Autodesk Inventor part; units mm, degrees
ref_plane "YZ Plane" through (0, 0, 0) normal (1, 0, 0) x (0, 1, 0)
ref_plane "XZ Plane" through (0, 0, 0) normal (0, 1, 0) x (-1, 0, 0)
ref_plane "XY Plane" through (0, 0, 0) normal (0, 0, 1) x (1, 0, 0)
sketch "Sketch1" plane through (0, 0, 0) normal (1, 0, 0) x (0, 1, 0)
  line L0 (0, 0) -> (11.43, 0)
  line L1 (11.43, 0) -> (11.43, -28.575)
  line L2 (11.43, -28.575) -> (0, -28.575)
  line L3 (0, -28.575) -> (0, 0)
  line L4 (0, 0) -> (8.255, 0)
  line L5 (8.255, 0) -> (8.255, -25.4)
  line L6 (8.255, -25.4) -> (0, -25.4)
  line L7 (0, -25.4) -> (0, 0)
  dimension "d0" = 11.43
  dimension "d1" = 28.575
  dimension "d2" = 8.255
  dimension "d3" = 25.4
extrude "Extrusion1" add sketch "Sketch1" along normal blind 19.05 contours L0 L1 L2 L3 L6 L5
sketch "Sketch2" plane through (0, 11.43, 0) normal (0, 1, 0) x (1, 0, 0)
  line L0 (0, 28.575) -> (0, 0)
  line L1 (0, 0) -> (19.05, 0)
  line L2 (19.05, 28.575) -> (19.05, 0)
  line L3 (0, 28.575) -> (19.05, 28.575)
  point P0 (0, 0)
  point P1 (4.7625, 6.35)
  point P2 (14.2875, 6.35)
  dimension "d6" = 9.525
  dimension "d7" = 4.7625
  dimension "d8" = 28.575
  dimension "d31" = 19.05
  dimension "d33" = 6.35
  dimension "d34" = 6.35
hole "Hole1" at (4.7625, 11.43, -6.35) at (14.2875, 11.43, -6.35) direction (0, -1, 0) diameter 3.429 end through all
sketch "Sketch3" plane through (0, 0, -25.4) normal (0, 0, 1) x (1, 0, 0)
  line L0 (0, 0) -> (0, 8.255)
  line L1 (19.05, 0) -> (0, 0)
  line L2 (19.05, 8.255) -> (19.05, 0)
  line L3 (0, 8.255) -> (19.05, 8.255)
  point P0 (0, 0)
  point P1 (4.7625, 4.1275)
  point P2 (14.2875, 4.1275)
  dimension "d20" = 9.525
  dimension "d21" = 4.7625
  dimension "d22" = 4.1275
  dimension "d23" = 4.1275
  dimension "d32" = 19.05
  dimension "d35" = 8.255
hole "Hole2" at (4.7625, 4.1275, -25.4) at (14.2875, 4.1275, -25.4) direction (0, 0, -1) diameter 3.81 end through all
properties part number "TensionerPlate4a" material "ABS Plastic"
Could you check a few things on this model? Use its own coordinates, in mm. A direction names the side the tool comes from. Coordinates: 2 decimals unless noted, no trailing zeros. Write each loop counter-clockwise with the first axis right and the second up, starting at its lowest first coordinate (ties: lowest second). Pieces come first, ordered by that corner, then holes. Notation, with made-up numbers: (38.25, 0) - (87.25, 0) arc R22 cw to (87.25, 35) - close; hole circle Ø1 at (57, -11.5). An arc over 180 degrees is marked (long way). Put each result on its own line as item: value. Start each with the question number.
Q1. Please list where these lines run through material, in increasing order: L1, parallel to X at y = 10.55, z = -6.35; L2, parallel to Z at x = 14.25, y = 8.5 (3 decimals); L3, parallel to Y at x = 9.5, z = -21.5 (3 decimals).
Q2. Thinking about a two-plate mould opening in Y: for faces 1 (the flat face through (19.05, 9, -17)), 2 (the flat face through (9, 11.43, -14)), 3 (the cylindrical face through (5.492, 2.368, -27.01)), which applies, pulls with the +Y half, pulls with the -Y half, needs draft (parallel to the pull), parting line crosses it, or undercut?
Q3. Which directions (+Z, -Z, +X, -X, +Y, -Y) give clear straight access to the entire face, cutting with the end or side of a thin tool? Please do faces 4 (the flat face through (9, 6, -28.575)), 5 (the flat face through (9, 4, -25.4)).
Q4. I want a section at A-A on z = -6.35. Write out the boundary of the cut face in (x, y) (3 decimals).
Q5. I want a section at C-C on y = 5. Write out the boundary of the cut face in (x, z) (3 decimals), plus the area to 3 significant figures.
Q6. I want a section at B-B on x = 3.75. Write out the boundary of the cut face in (y, z) (3 decimals), plus the area to 3 significant figures.
Q7. I want a section at D-D on y = 9.75. Count the separate pieces of the cut face and the enclosed holes in it, plus the area to 3 significant figures.
Q8. I'm going to push flat-ended pins straight in: P1, Ø2, axis at x = 14, z = -7.5, coming from the +Y side; P2, Ø2, axis at x = 12.5, y = 2.5, coming from the +Z side; P3, Ø2.5, axis at x = 4.76, y = 4.13, coming from the -Z side; P4, Ø6, axis at x = 14.5, z = -3.5, coming from the -Y side (3 decimals). Where does each tip first touch, or does it pass through?
Checks:
1. L1: 0 to 3.05, 6.48 to 12.57, 16 to 19.05
1. L2: -28.575 to -8.064, -4.636 to 0
1. L3: 8.255 to 11.43
2. face 1: needs draft
2. face 2: pulls with the +Y half
2. face 3: undercut
3. face 4: -Z, +X, -X, +Y, -Y
3. face 5: +Z, +X, -X, -Y
4. outline: (0, 8.255) - (3.048, 8.255) - (3.048, 11.43) - (0, 11.43) - close; (6.477, 8.255) - (12.573, 8.255) - (12.573, 11.43) - (6.477, 11.43) - close; (16.002, 8.255) - (19.05, 8.255) - (19.05, 11.43) - (16.002, 11.43) - close
5. outline: (0, -28.575) - (3.069, -28.575) - (3.069, -25.4) - (0, -25.4) - close; (6.456, -28.575) - (12.594, -28.575) - (12.594, -25.4) - (6.456, -25.4) - close; (15.981, -28.575) - (19.05, -28.575) - (19.05, -25.4) - (15.981, -25.4) - close
5. area: 39.0 mm²
6. outline: (0, -28.575) - (2.514, -28.575) - (2.514, -25.4) - (0, -25.4) - close; (5.741, -28.575) - (11.43, -28.575) - (11.43, -7.734) - (8.255, -7.734) - (8.255, -25.4) - (5.741, -25.4) - close; (8.255, -4.966) - (11.43, -4.966) - (11.43, 0) - (8.255, 0) - close
6. area: 97.9 mm²
7. separate pieces: 1
7. enclosed holes: 2
7. area: 526 mm²
8. P1: y = 11.43
8. P2: z = -25.4
8. P3: through
8. P4: y = 8.255
